Could you check a few things on this model? Use its own coordinates, in mm. A direction names the side the tool comes from. Give positions to 0.01 mm unless a question says otherwise; leave off trailing zeros. Order: outer loops, then holes, each group sorted by start corner. A loop starts at its lowest first (then second) coordinate and runs counter-clockwise, first axis right, second up. Notation, with made-up numbers: (83, 44) -> (111, 44) arc R23 cw to (111, 62) -> close; hole circle Ø11 at (68.25, 45.5). An arc over 180 degrees is marked (long way). Answer as CSV lines item,"result". Start each with the question number.
(1) Will these pins go through, and if not, where does the flat tip stop? pin 1 Ø3 at (x, z) = (8.5, 0.5) entering from -Y; pin 2 Ø4 at (x, y) = (-7.5, -4.5) entering from -Z; pin 3 Ø1 at (x, z) = (-4.5, 0.5) entering from +Y; pin 4 Ø1.6 at (x, z) = (-2.5, 10.5) entering from +Y.
(2) I need wall thicknesses on L1, parallel to Z at x = 10, y = -0.55; L2, parallel to Y at x = 6.5, z = -11; L3, parallel to Y at x = -2.75, z = 1. Which ranges of each line are inside material? Lowest first, please.
(3) I want a section at C-C (z = 4.75). Please give me the cut outline in (x, y), plus the area to 4 significant figures.
(4) I want a section at B-B (z = -10.5). Please give me the cut outline in (x, y), plus the area to 3 significant figures.
(5) I want a section at D-D (x = -0.75). Please give me the cut outline in (y, z), plus the area to 3 significant figures.
(6) On a 3-axis mill with a long thin cutter (end or side, diameter ignored), from which of +Z, -Z, +X, -X, +Y, -Y can I reach the whole of each face in a straight line? I mean faces 4 (the face through (-6.5, 1, 0)), 5 (the face through (-3, -5.9, 0)), 6 (the face through (-7, -3, 0)), 7 (the face through (-9, 1, 10)), 8 (the face through (-3, -3, -4.25)). Say none if no direction works.
(7) We'd pull the mould along Z, two halves only. Please class faces 1 (the face through (9.263, -0.456, 11.176)), 2 (the face through (1.5, -3, 0)), 3 (the face through (-3, -3, 4.25)): released by +Z, released by -Z, zero draft, split by the parting line, or undercut.
(8) I want a section at A-A (x = 10). Please give me the cut outline in (y, z).
```python
from build123d import *

# Parameters (mm, degrees)
F0_W     = 24
F0_H     = 25
F1_DEPTH = 0.9
F2_R     = 1
F3_W     = 8.5
F3_H     = 8.5
F4_DEPTH = 5
F5_R     = 1
F6_DEPTH = 0.901
F7_W     = 5.5
F7_H     = 20
F8_DEPTH = 2.5


with BuildPart() as f1:
    # F0 (on Front) → F1 (new body)
    with BuildSketch(Plane.XZ):
        Rectangle(F0_W, F0_H)
    extrude(amount=F1_DEPTH)

    # F2
    f2_edges = [f1.edges().sort_by_distance(p)[0] for p in [
        (12, -0.45, 12.5),
        (12, -0.45, -12.5),
        (-12, -0.45, -12.5),
        (-12, -0.45, 12.5),
    ]]
    fillet(f2_edges, radius=F2_R)

    # F3 (on face) → F4 (join)
    with BuildSketch(Plane.XZ.offset(0.9)):
        with Locations((-2.75, 0)):
            Rectangle(F3_W, F3_H)
    extrude(amount=F4_DEPTH)

    # F5 (on face) → F6 (cut, through all)
    with BuildSketch(Plane.XZ.offset(0.9)):
        with Locations((10, 10.5)):
            Circle(F5_R)
        with Locations((-2.5, 10.5)):
            Circle(F5_R)
        with Locations((-2.5, -10.5)):
            Circle(F5_R)
        with Locations((10, -10.5)):
            Circle(F5_R)
    extrude(amount=-F6_DEPTH, mode=Mode.SUBTRACT)

    # F7 (on face) → F8 (join)
    with BuildSketch(Plane(origin=(0, 0, 0), x_dir=(-1, 0, 0), z_dir=(0, 1, 0))):
        with Locations((9.25, 0)):
            Rectangle(F7_W, F7_H)
    extrude(amount=F8_DEPTH)


solid = f1.part
```
Final values:
1,pin 1,"y = -0.9"
1,pin 2,"z = -4.25"
1,pin 3,"y = 0"
1,pin 4,"through"
2,L1,"-12.5 to -11.5, -9.5 to 9.5, 11.5 to 12.5"
2,L2,"-0.9 to 0"
2,L3,"-5.9 to 0"
3,outline,"(-12, -0.9) -> (12, -0.9) -> (12, 0) -> (-6.5, 0) -> (-6.5, 2.5) -> (-12, 2.5) -> close"
3,area,"35.35 mm²"
4,outline,"(-12, -0.9) -> (-3.5, -0.9) -> (-3.5, 0) -> (-12, 0) -> close; (-1.5, -0.9) -> (9, -0.9) -> (9, 0) -> (-1.5, 0) -> close; (11, -0.9) -> (12, -0.9) -> (12, 0) -> (11, 0) -> close"
4,area,"18.0 mm²"
5,outline,"(-5.9, -4.25) -> (-0.9, -4.25) -> (-0.9, -12.5) -> (0, -12.5) -> (0, 12.5) -> (-0.9, 12.5) -> (-0.9, 4.25) -> (-5.9, 4.25) -> close"
5,area,"65.0 mm²"
6,face 4,"+Z, -Z, +X, +Y"
6,face 5,"+Z, -Z, +X, -X, -Y"
6,face 6,"+Z, -Z, -X, -Y"
6,face 7,"+Z, +X, -X, +Y"
6,face 8,"-Z, +X, -X, -Y"
7,face 1,"undercut"
7,face 2,"zero draft"
7,face 3,"released by +Z"
8,outline,"(-0.9, -12.5) -> (0, -12.5) -> (0, -11.5) -> (-0.9, -11.5) -> close; (-0.9, -9.5) -> (0, -9.5) -> (0, 9.5) -> (-0.9, 9.5) -> close; (-0.9, 11.5) -> (0, 11.5) -> (0, 12.5) -> (-0.9, 12.5) -> close"
